Could you check a few things on this model? Use its own coordinates, in mm. Face numbers are marked on the shaded views. A direction names the side the tool comes from. Give positions to 0.01 mm unless a question says otherwise; leave off trailing zeros. Write each loop counter-clockwise with the first axis right and the second up, starting at its lowest first coordinate (ties: lowest second). Pieces come first, ordered by that corner, then holes. Notation, with made-up numbers: (68, -12) - (84, -12) arc R13 cw to (84, -5) - close; hole circle Ø4 at (36, 75). An arc over 180 degrees is marked (long way). Write item = value, one per line.
from build123d import *

# Parameters (mm, degrees)
PAD_DEPTH       = 20
POCKET004_DEPTH = 10
POCKET001_DEPTH = 17.4
SKETCH004_R     = 2.15
POCKET003_DEPTH = 15
SKETCH007_R     = 2.15
POCKET_DEPTH    = 37
SKETCH008_R     = 2.15
POCKET005_DEPTH = 10
SKETCH005_R     = 12.1
SKETCH005_R_2   = 2
PAD001_DEPTH    = 4
SKETCH009_R     = 7.5
PAD002_DEPTH    = 8
SKETCH010_R     = 2.15
POCKET006_DEPTH = 8


with BuildPart() as part:
    # Sketch → Pad (new body)
    with BuildSketch(Plane.XZ):
        with BuildLine():
            Line((4.0389999215, 42.5749876661), (2.65554232, 42.7947220429))
            ThreePointArc((2.9065240645, 44.3749144882), (1.9909369697, 43.7103091378), (2.65554232, 42.7947220429))
            Line((2.9065240645, 44.3749144882), (5.0304287832, 44.0375749995))
            Line((5.0304287832, 44.0375749995), (5.0304287832, 45.6803340803))
            ThreePointArc((6.6304287832, 45.6803340803), (5.8304287832, 46.4803340803), (5.0304287832, 45.6803340803))
            Line((6.6304287832, 45.6803340803), (6.6304287832, 44.1673826739))
            Line((6.6304287832, 44.1673826739), (8.4415552878, 45.4119716817))
            Line((8.4415552878, 45.4119716817), (9.4478356401, 46.1368713386))
            ThreePointArc((10.3621773687, 44.8642380551), (10.5421249478, 45.9583016271), (9.4478356401, 46.1368713386))
            Line((10.3621773687, 44.8642380551), (7.8490460164, 43.0634365917))
            Line((7.8490460164, 43.0634365917), (5.6389999215, 41.5447138136))
            Line((5.6389999215, 41.5447138136), (7.0548889855, 39.4843113873))
            Line((7.0548889855, 39.4843113873), (12.3295191968, 43.1089873912))
            Line((12.3295191968, 43.1089873912), (38.948233601, 4.3734217768))
            Line((134.8805705695, 70.297216599), (38.948233601, 4.3734217768))
            Line((119.305790865, 92.9616432883), (134.8805705695, 70.297216599))
            Line((134.9648493048, 103.722400175), (119.305790865, 92.9616432883))
            Line((142.0442946251, 93.4203880435), (134.9648493048, 103.722400175))
            Line((142.0442946251, 93.4203880435), (153.0527823524, 77.9305340853))
            Line((153.0527823524, 77.9305340853), (165.0024035036, 60.5414398134))
            Line((165.0024035036, 60.5414398134), (260.687492181, 126.2953279479))
            Line((260.687492181, 126.2953279479), (237.9766315936, 159.3441828657))
            Line((219.8532515738, 185.7173339224), (237.9766315936, 159.3441828657))
            Line((225.1278817851, 189.3420099263), (219.8532515738, 185.7173339224))
            Line((223.7119927211, 191.4024123526), (225.1278817851, 189.3420099263))
            Line((218.4373625097, 187.7777363487), (223.7119927211, 191.4024123526))
            Line((218.4373625097, 187.7777363487), (217.5311935087, 189.0963939015))
            Line((217.5311935087, 189.0963939015), (221.3847855834, 191.7445459354))
            Line((221.3847855834, 191.7445459354), (219.3797100852, 192.170938972))
            ThreePointArc((219.6293167368, 193.3446921486), (218.9176368227, 192.882618886), (219.3797100852, 192.170938972))
            Line((219.6293167368, 193.3446921486), (221.2499182947, 193.0000601284))
            Line((221.2499182947, 193.0000601284), (222.3399490261, 195.3337880811))
            ThreePointArc((223.4271977541, 194.8259591695), (223.1374878459, 195.6234979893), (222.3399490261, 195.3337880811))
            Line((223.4271977541, 194.8259591695), (222.4600969226, 192.7554209925))
            Line((222.4600969226, 192.7554209925), (225.3603146621, 192.5351236039))
            Line((225.3603146621, 192.5351236039), (227.2063997814, 189.8486996774))
            Line((227.2063997814, 189.8486996774), (225.1628423907, 186.8509880341))
            Line((225.1628423907, 186.8509880341), (229.8798569494, 185.6901424243))
            ThreePointArc((229.5930959709, 184.5249093398), (230.3190930024, 184.9641453928), (229.8798569494, 185.6901424243))
            Line((229.5930959709, 184.5249093398), (227.4496707489, 185.0524009826))
            Line((227.4496707489, 185.0524009826), (226.9444544706, 182.6614258938))
            ThreePointArc((225.771548638, 182.6560117607), (226.3601860514, 182.1854742091), (226.9444544706, 182.6614258938))
            Line((225.771548638, 182.6560117607), (226.2739055744, 185.0334547935))
            Line((226.2739055744, 185.0334547935), (223.7978510454, 183.3319335348))
            Line((223.7978510454, 183.3319335348), (226.0066379853, 180.1177057498))
            Line((226.0066379853, 180.1177057498), (232.1878452642, 184.365372942))
            Line((266.2495585655, 125.2641065683), (232.1878452642, 184.365372942))
            Line((244.0796284586, 110.0291402391), (266.2495585655, 125.2641065683))
            Line((290.6340608845, 42.2831084623), (244.0796284586, 110.0291402391))
            Line((294.2587368885, 37.008478251), (290.6340608845, 42.2831084623))
            Line((296.3191393148, 38.424367315), (294.2587368885, 37.008478251))
            Line((292.4602624187, 44.0398067738), (296.3191393148, 38.424367315))
            Line((292.4602624187, 44.0398067738), (293.7789199715, 44.9459757748))
            Line((293.7789199715, 44.9459757748), (296.6206071991, 40.810751196))
            Line((296.6206071991, 40.810751196), (297.0910989584, 42.7718237934))
            ThreePointArc((298.2579860864, 42.4918694569), (297.8145196907, 43.2152901891), (297.0910989584, 42.7718237934))
            Line((298.2579860864, 42.4918694569), (297.7424907939, 40.3432161125))
            Line((297.7424907939, 40.3432161125), (300.1208515514, 39.8397804262))
            ThreePointArc((299.8723496236, 38.6657928658), (300.5835943677, 39.1285356821), (300.1208515514, 39.8397804262))
            Line((299.8723496236, 38.6657928658), (297.7654069562, 39.1117765647))
            Line((297.7654069562, 39.1117765647), (296.952983451, 36.4332286099))
            Line((296.952983451, 36.4332286099), (295.3914481397, 35.36015631))
            Line((295.3914481397, 35.36015631), (291.8734642457, 36.02124884))
            Line((291.8734642457, 36.02124884), (290.5930300808, 32.2088535913))
            ThreePointArc((289.4324911908, 32.3007970199), (289.9768664604, 31.8017577275), (290.5930300808, 32.2088535913))
            Line((289.4324911908, 32.3007970199), (290.1466686614, 34.4272060697))
            Line((290.1466686614, 34.4272060697), (287.5314050616, 35.2037645635))
            ThreePointArc((287.8729844966, 36.3541225467), (287.1270157875, 35.9497332726), (287.5314050616, 35.2037645635))
            Line((287.8729844966, 36.3541225467), (290.0582057564, 35.7052578853))
            Line((290.0582057564, 35.7052578853), (288.248660497, 38.3385089907))
            Line((288.248660497, 38.3385089907), (285.034432712, 36.1297220508))
            Line((285.034432712, 36.1297220508), (289.2820999041, 29.9485147719))
            Line((289.2820999041, 29.9485147719), (228.6149276864, -5.1892742181))
            Line((37.9174947707, -1.1893468138), (228.6149276864, -5.1892742181))
            Line((9.1698866415, 31.1095406492), (37.9174947707, -1.1893468138))
            Line((15.3510939204, 35.3572078414), (9.1698866415, 31.1095406492))
            Line((13.1423069804, 38.5714356264), (15.3510939204, 35.3572078414))
            Line((10.6193023838, 36.8376507253), (13.1423069804, 38.5714356264))
            Line((12.456789603, 36.8376507253), (10.6193023838, 36.8376507253))
            ThreePointArc((12.456789603, 35.2376507253), (13.256789603, 36.0376507253), (12.456789603, 36.8376507253))
            Line((10.207394012, 35.2376507253), (12.456789603, 35.2376507253))
            Line((10.207394012, 33.9421349105), (10.207394012, 35.2376507253))
            ThreePointArc((8.607394012, 33.9421349105), (9.407394012, 33.1421349105), (10.207394012, 33.9421349105))
            Line((8.607394012, 37.2723114812), (8.607394012, 33.9421349105))
            Line((5.4065670445, 38.351600136), (8.607394012, 37.2723114812))
            Line((4.0389999215, 40.3416844512), (5.4065670445, 38.351600136))
            Line((4.0389999215, 40.3416844512), (4.0389999215, 42.5749876661))
        make_face()
        Polygon((149.7561384703, 75.6651115828), (163.971182124, 54.9793734288), (179.795072758, 65.8534014407), (225.8253519656, -1.1298823283), (43.5671319438, 2.6930304282), align=None, mode=Mode.SUBTRACT)
        Polygon((247.6318069807, 78.3748825832), (199.00630972, 44.9599006716), (229.646149066, 0.3727921664), (281.0213223864, 29.7864441936), align=None, mode=Mode.SUBTRACT)
    extrude(amount=PAD_DEPTH)

    # Sketch006 → Pocket004 (cut)
    with BuildSketch(Plane.XZ):
        Polygon((291.8154691607, 43.5532983952), (229.6803031775, 0.323320239), (193.027696, 53.659792), (184.530685, 47.990654), (178.024719, 57.651035), (186.3396484214, 63.3921652896), (183.0916284776, 68.1186482583), (245.422424, 110.825737), align=None)
    extrude(amount=POCKET004_DEPTH, mode=Mode.SUBTRACT)

    # Sketch002 → Pocket001 (cut)
    with BuildSketch(Plane.XZ):
        Polygon((240.839386, 107.681338), (254.396576976, 87.8772330508), (208.1871169974, 56.2436147234), (194.629852, 76.047669), align=None)
    extrude(amount=POCKET001_DEPTH, mode=Mode.SUBTRACT)

    # Sketch004 (on DatumPlane) → Pocket003 (cut)
    with BuildSketch(Plane(origin=(217.1470694031, 0, 149.2214127365), x_dir=(-0.5663556256, 0, 0.8241609705), z_dir=(0.8241609705, 0, 0.5663556256))):
        with Locations((-123.5, 13.5)):
            Circle(SKETCH004_R)
        with Locations((-93, 13.5)):
            Circle(SKETCH004_R)
        with Locations((-108.25, 13.5)):
            Circle(SKETCH004_R)
        with Locations((-77.75, 13.5)):
            Circle(SKETCH004_R)
    extrude(amount=-POCKET003_DEPTH, mode=Mode.SUBTRACT)

    # Sketch007 (on DatumPlane) → Pocket (cut)
    with BuildSketch(Plane(origin=(-5.1231693546, 0, 7.455238434), x_dir=(-0.8241609705, 0, -0.5663556256), z_dir=(-0.5663556256, 0, 0.8241609705))):
        with Locations((-160.5, 10)):
            Circle(SKETCH007_R)
    extrude(amount=-POCKET_DEPTH, mode=Mode.SUBTRACT)

    # Sketch008 (on DatumPlane) → Pocket005 (cut)
    with BuildSketch(Plane(origin=(28.496623251, 0, 19.5826100321), x_dir=(-0.5663556256, 0, 0.8241609705), z_dir=(0.8241609705, 0, 0.5663556256))):
        with Locations((-122.5, 13.5)):
            Circle(SKETCH008_R)
        with Locations((-92, 13.5)):
            Circle(SKETCH008_R)
    extrude(amount=-POCKET005_DEPTH, mode=Mode.SUBTRACT)

    # Sketch005 (on DatumPlane) → Pad001 (join)
    with BuildSketch(Plane.XZ.offset(20)):
        Polygon((5.6390093024, 41.5438867756), (7.0549059293, 39.4834895465), (13.31004, 39.773029), (37.917178458, -1.1893531666), (228.649104, -5.2387525299), (287.152954, 30.335571), (283.599121, 36.427879), (290.421173, 40.857933), (242.328964, 110.216705), (262.12204, 125.860641), (222.003006, 184.166046), (225.1273486637, 189.3419885374), (223.7114520368, 191.4023857666), (218.756056001, 189.9384309091), (114.4490881489, 118.7444485703), (124.6435438626, 103.9095885203), (122.8303943009, 102.6635994887), (112.6359385872, 117.4984595386), (8.4415504736, 45.4111549307), align=None)
        with Locations((141.5496774667, 14.6144979084)):
            Circle(SKETCH005_R, mode=Mode.SUBTRACT)
        with Locations((153.6381766572, 24.0175512593)):
            Circle(SKETCH005_R_2, mode=Mode.SUBTRACT)
        with Locations((129.4611782762, 5.2114445574)):
            Circle(SKETCH005_R_2, mode=Mode.SUBTRACT)
        Polygon((118.9759479588, 92.734690012), (135.2942940138, 103.948591297), (124.1936644589, 120.1021055736), (122.2156831189, 118.7428448118), (132.0703236421, 104.4024800969), (119.7079402671, 95.9071003355), (109.8532997439, 110.2474650504), (107.8753184039, 108.8882042886), align=None, mode=Mode.SUBTRACT)
    extrude(amount=-PAD001_DEPTH)

    # Sketch009 (on DatumPlane) → Pad002 (join)
    with BuildSketch(Plane(origin=(26.9325590555, 0, -39.1922724975), x_dir=(0.8241609705, 0, 0.5663556256), z_dir=(0.5663556256, 0, -0.8241609705))):
        with Locations((280, 10)):
            Circle(SKETCH009_R)
    extrude(amount=-PAD002_DEPTH)

    # Sketch010 (on DatumPlane) → Pocket006 (cut)
    with BuildSketch(Plane(origin=(26.9325590555, 0, -39.1922724975), x_dir=(0.8241609705, 0, 0.5663556256), z_dir=(0.5663556256, 0, -0.8241609705))):
        with Locations((280, 10)):
            Circle(SKETCH010_R)
    extrude(amount=-POCKET006_DEPTH, mode=Mode.SUBTRACT)


solid = part.part
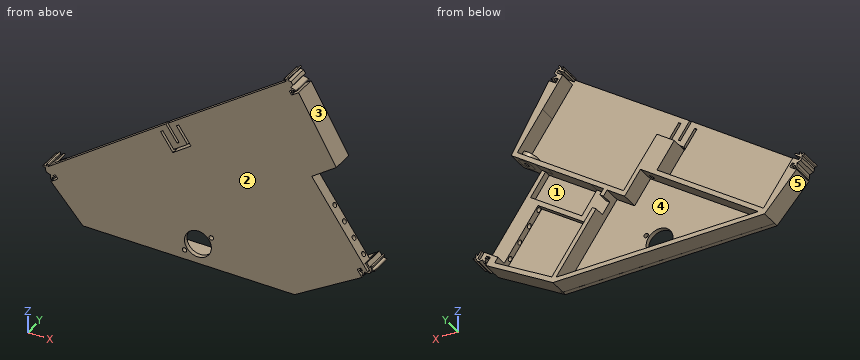
1. If we section it at C-C, the plane x = 22: Please give me the cut outline in (y, z).
Filled sheet:
outline = (-20, 16.69) - (0, 16.69) - (0, 29.04) - (-16, 29.04) - (-16, 54.79) - (-20, 54.79) - close
2. Which directions (+Z, -Z, +X, -X, +Y, -Y) give clear straight access to the entire face, cutting with the end or side of a thin tool? Please do the marked faces 4 and 5.
Filled sheet:
face_4 = +Y
face_5 = -Z, -X, +Y, -Y
3. Thinking about a two-plate mould opening in X: for the marked faces 1, 2 and 3, which applies, pulls with the +X half, pulls with the -X half, needs draft (parallel to the pull), parting line crosses it, or undercut?
Filled sheet:
face_1 = undercut
face_2 = needs draft
face_3 = pulls with the +X half
4. I need wall thicknesses on line 1 (X direction, y = -9, z = 70.5); line 2 (X direction, y = -15, z = 66); line 3 (X direction, y = -8.5, z = 21). Which ranges of each line are inside material? Lowest first, please.
Filled sheet:
line_1 = 134.74 to 142.24, 153.31 to 158.16, 179.49 to 186.57
line_2 = 128.63 to 135.69, 156.4 to 161.25, 172.95 to 201.51, 222.44 to 229.62, 256.14 to 257.53, 262.97 to 274.34
line_3 = 18.17 to 27.52, 63.14 to 70.21, 210.62 to 215.47, 265.67 to 273.83
5. If we section it at B-B, the plane z = 145.5: Please give me the cut outline in (x, y), and give its area (3 significant figures).
Filled sheet:
outline = (153.65, -20) - (254.59, -20) - (254.59, 0) - (247.49, 0) - (247.49, -16) - (153.65, -16) - close
area = 517 mm2
6. For pin 1 (6 mm diameter, centred on y = -16.5, z = 133.5, fed in from -X); pin 2 (1 mm diameter, centred on x = 160, z = 85, fed in from +Y); pin 3 (1 mm diameter, centred on x = 263.5, y = -2, fed in from -Z), each with a flat end and sliding along its axis, tell me the tip position at first contact or that it passes through.
Filled sheet:
pin_1 = 131.67
pin_2 = -16
pin_3 = 14.73
